from build123d import *

# Parameters (mm, degrees)
SKETCH_1_W          = 42
SKETCH_1_H          = 42
EXTRUDE_1_DEPTH     = 33
CHAMFER_1_SIZE      = 10
SKETCH_2_W          = 42.3
SKETCH_2_H          = 42.3
EXTRUDE_2_DEPTH     = 7.5
SKETCH_3_W          = 42.3
SKETCH_3_H          = 42.3
EXTRUDE_3_DEPTH     = 7.5
CHAMFER_2_SIZE      = 5
SKETCH_4_R          = 1.5
CUT_EXTRUDE_1_DEPTH = 4.5
SKETCH_5_R          = 11
SKETCH_5_R_2        = 3.75
EXTRUDE_4_DEPTH     = 2
SKETCH_6_R          = 2.5
EXTRUDE_5_DEPTH     = 24
CUT_EXTRUDE_START   = -19
CUT_EXTRUDE_2_DEPTH = 19
CHAMFER_3_SIZE      = 0.5
EXTRUDE_6_DEPTH     = 2.5
FILLET_1_R          = 1
EXTRUDE_7_DEPTH     = 5
EXTRUDE_8_DEPTH     = 9
CHAMFER_4_SIZE      = 2.5


with BuildPart() as part:
    # 草图1 → 凸台-拉伸1 (new body)
    with BuildSketch(Plane.XY):
        Rectangle(SKETCH_1_W, SKETCH_1_H)
    extrude(amount=EXTRUDE_1_DEPTH)

    # 倒角1
    chamfer_1_edges = [part.edges().sort_by_distance(p)[0] for p in [
        (21, -21, 16.5),
        (-21, -21, 16.5),
        (-21, 21, 16.5),
        (21, 21, 16.5),
    ]]
    chamfer(chamfer_1_edges, length=CHAMFER_1_SIZE)

    # 草图2 → 凸台-拉伸2 (add)
    with BuildSketch(Plane.XY.offset(33)):
        Rectangle(SKETCH_2_W, SKETCH_2_H)
    extrude(amount=EXTRUDE_2_DEPTH)

    # 草图3 → 凸台-拉伸3 (add)
    with BuildSketch(Plane(origin=(0, 0, 0), x_dir=(-1, 0, 0), z_dir=(0, 0, -1))):
        Rectangle(SKETCH_3_W, SKETCH_3_H)
    extrude(amount=EXTRUDE_3_DEPTH)

    # 倒角2
    chamfer_2_edges = [part.edges().sort_by_distance(p)[0] for p in [
        (21.15, -21.15, 36.75),
        (21.15, 21.15, 36.75),
        (-21.15, 21.15, 36.75),
        (-21.15, -21.15, 36.75),
        (-21.15, -21.15, -3.75),
        (-21.15, 21.15, -3.75),
        (21.15, 21.15, -3.75),
        (21.15, -21.15, -3.75),
    ]]
    chamfer(chamfer_2_edges, length=CHAMFER_2_SIZE)

    # 草图4 → 切除-拉伸1 (cut)
    with BuildSketch(Plane(origin=(0, 0, -7.5), x_dir=(-1, 0, 0), z_dir=(0, 0, -1))):
        with Locations((-15.5, 15.5)):
            Circle(SKETCH_4_R)
        with Locations((15.5, 15.5)):
            Circle(SKETCH_4_R)
        with Locations((15.5, -15.5)):
            Circle(SKETCH_4_R)
        with Locations((-15.5, -15.5)):
            Circle(SKETCH_4_R)
    extrude(amount=-CUT_EXTRUDE_1_DEPTH, mode=Mode.SUBTRACT)

    # 草图5 → 凸台-拉伸4 (add)
    with BuildSketch(Plane(origin=(0, 0, -7.5), x_dir=(-1, 0, 0), z_dir=(0, 0, -1))):
        Circle(SKETCH_5_R)
        Circle(SKETCH_5_R_2, mode=Mode.SUBTRACT)
    extrude(amount=EXTRUDE_4_DEPTH)

    # 草图6 → 凸台-拉伸5 (add)
    with BuildSketch(Plane(origin=(0, 0, -7.5), x_dir=(-1, 0, 0), z_dir=(0, 0, -1))):
        Circle(SKETCH_6_R)
    extrude(amount=EXTRUDE_5_DEPTH)

    # 草图7 → 切除-拉伸2 (cut)
    with BuildSketch(Plane(origin=(0, 0, -31.5), x_dir=(-1, 0, 0), z_dir=(0, 0, -1)).offset(CUT_EXTRUDE_START)):
        with BuildLine():
            Line((2, 1.5), (-2, 1.5))
            ThreePointArc((-2, 1.5), (0, 2.5), (2, 1.5))
        make_face()
    extrude(amount=CUT_EXTRUDE_2_DEPTH, mode=Mode.SUBTRACT)

    # 倒角3
    chamfer_3_edges = [part.edges().sort_by_distance(p)[0] for p in [
        (0.790569415, -2.371708245, -31.5),
    ]]
    chamfer(chamfer_3_edges, length=CHAMFER_3_SIZE)

    # 草图8 → 凸台-拉伸6 (add)
    with BuildSketch(Plane.XY.offset(40.5)):
        Polygon((0, 21.15), (-8, 21.15), (-8, 25.15), (8, 25.15), (8, 21.15), align=None)
    extrude(amount=-EXTRUDE_6_DEPTH)

    # 圆角1
    fillet_1_edges = [part.edges().sort_by_distance(p)[0] for p in [
        (-12.075, 21.15, 40.5),
        (8, 23.15, 40.5),
        (0, 25.15, 40.5),
        (-8, 23.15, 40.5),
        (0, -21.15, 40.5),
        (-21.15, 0, 40.5),
        (21.15, 0, 40.5),
        (12.075, 21.15, 40.5),
        (-18.65, 18.65, 40.5),
        (18.65, 18.65, 40.5),
        (18.65, -18.65, 40.5),
        (-18.65, -18.65, 40.5),
    ]]
    fillet(fillet_1_edges, radius=FILLET_1_R)

    # 草图9 → 凸台-拉伸7 (add)
    with BuildSketch(Plane(origin=(0, 21.15, 0), x_dir=(1, 0, 0), z_dir=(0, 1, 0))):
        Polygon((7.9, -33), (5, -33), (5, -33.5), (7.5, -33.5), (7.5, -37.5), (-7.5, -37.5), (-7.5, -33.5), (-5, -33.5), (-5, -33), (-7.9, -33), (-7.9, -38), (7.9, -38), align=None)
    extrude(amount=EXTRUDE_7_DEPTH)

    # 草图10 → 凸台-拉伸8 (add)
    with BuildSketch(Plane.XY.offset(40.5)):
        Polygon((-7, 20.15), (-15.735786438, 20.15), (-20.15, 15.735786438), (-20.15, -15.735786438), (-15.735786438, -20.15), (15.735786438, -20.15), (20.15, -15.735786438), (20.15, 15.735786438), (15.735786438, 20.15), (7, 20.15), (7, 24.15), (-7, 24.15), align=None)
    extrude(amount=EXTRUDE_8_DEPTH)

    # 倒角4
    # the kernel refuses this chamfer: 2.5 mm, written as the material it adds along each edge
    with BuildSketch(Plane(origin=(0, 0, -7.5), x_dir=(-1, 0, 0), z_dir=(0, -1, 0))) as chamfer_4_piece_1:
        Polygon((2.5 + CHAMFER_4_SIZE, 0), (2.5, CHAMFER_4_SIZE), (2.5, 0), align=None)
    revolve(axis=Axis((0, 0, -7.5), (0, 0, -1)))


solid = part.part
CAD build for the part. Positions are in the model's coordinates, mm. A direction names the side the tool comes from. Coordinates: 2 decimals unless noted, no trailing zeros. Write each loop counter-clockwise with the first axis right and the second up, starting at its lowest first coordinate (ties: lowest second). Pieces come first, ordered by that corner, then holes. Notation, with made-up numbers: (88.25, 87.5) - (99.25, 87.5) arc R20 cw to (99.25, 114.5) - close; hole circle Ø11 at (84.5, 46). An arc over 180 degrees is marked (long way). Use a Markdown table: item, result. Add a question column.
Item 1: Flat gauge pins, fed straight in: pin 1 (4.5 mm diameter, centred on y = 23.5, z = 34.5, fed in from -X); pin 2 (5.5 mm diameter, centred on y = 25, z = 36, fed in from +X); pin 3 (8 mm diameter, centred on x = 3, z = 9.5, fed in from +Y). Where does each tip first touch, or does it go through?
Item 2: Mould opens along Z. For faces 4 (the face through (21, 0, 16)), 5 (the face through (-18.7, 18.6, -3.7)), 6 (the face through (-16, 17, 0)), 7 (the face through (-15, -15, -3)) say: pulls with the +Z half, pulls with the -Z half, needs draft (parallel to the pull), parting line crosses it, or undercut.
Item 3: Drill centre lines: L1, parallel to Y at x = 15.5, z = -6.3; L2, parallel to Y at x = -15, z = -6. Where is each one in solid material? Low to high. Write a range as from..to.
Item 4: Band-saw the part on D-D, the plane y = -12. Give the cut face in (x, z).
Item 5: Band-saw the part on C-C, the plane x = 13. Give the cut face in (y, z).
Item 6: Band-saw the part on B-B, the plane z = 29. Give the cut face in (x, y).
Item 7: 3-axis set-ups, long thin cutter, end or side, ignore diameter. For faces 1 (the face through (17, -15.43, -5.28)), 2 (the face through (0, 24.15, 45)), 3 (the face through (17.912, -17.974, 44.937)): which of +Z, -Z, +X, -X, +Y, -Y reach the whole face in a straight line?
Numbers:
| question | item | result |
|---|---|---|
| 1 | pin 1 | x = -7.9 |
| 1 | pin 2 | x = 8 |
| 1 | pin 3 | y = 21 |
| 2 | face 4 | undercut |
| 2 | face 5 | needs draft |
| 2 | face 6 | undercut |
| 2 | face 7 | pulls with the -Z half |
| 3 | L1 | -21.15..-17, -14..14, 17..21.15 |
| 3 | L2 | -21.15..-16.91, -14.09..14.09, 16.91..21.15 |
| 4 | outline | (-21.15, -7.5) - (21.15, -7.5) - (21.15, 0) - (20, 0) - (20, 33) - (21.15, 33) - (21.15, 39.5) arc R1 ccw to (20.15, 40.5) - (20.15, 49.5) - (-20.15, 49.5) - (-20.15, 40.5) arc R1 ccw to (-21.15, 39.5) - (-21.15, 33) - (-20, 33) - (-20, 0) - (-21.15, 0) - close |
| 5 | outline | (-21.15, -7.5) - (21.15, -7.5) - (21.15, 0) - (19, 0) - (19, 33) - (21.15, 33) - (21.15, 39.5) arc R1 ccw to (20.15, 40.5) - (20.15, 49.5) - (-20.15, 49.5) - (-20.15, 40.5) arc R1 ccw to (-21.15, 39.5) - (-21.15, 33) - (-19, 33) - (-19, 0) - (-21.15, 0) - close |
| 6 | outline | (-21, -11) - (-11, -21) - (11, -21) - (21, -11) - (21, 11) - (11, 21) - (-11, 21) - (-21, 11) - close |
| 7 | face 1 | -Z |
| 7 | face 2 | +Z, +X, -X, +Y |
| 7 | face 3 | +Z, +X, -Y |
